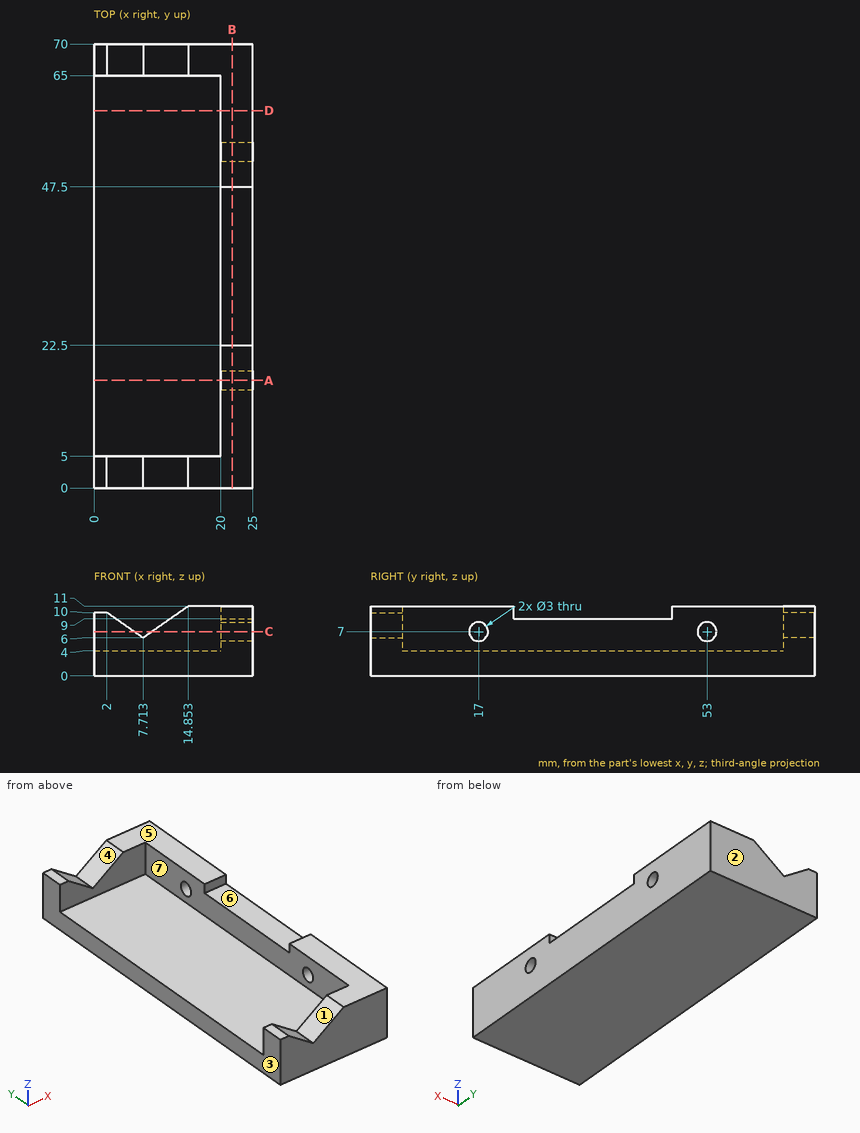
Verification items for this drawing (mm, ordinates from the low corner). A direction names the side the tool comes from. Coordinates: 2 decimals unless noted, no trailing zeros. Write each loop counter-clockwise with the first axis right and the second up, starting at its lowest first coordinate (ties: lowest second). Pieces come first, ordered by that corner, then holes. Notation, with made-up numbers: M 4.5,-18 L 29.5,-18 A30 cw 29.5,12 Z; hole C -22.75,24 d6. An arc over 180 degrees is marked long. One line per item, written item: value. Start each with the question number.
(1) Sectioned sample at A-A, the plane y = 17. Enter the section's corners in (x, z).
(2) Scan lines: line 1 along Y through (x, z) = (21, 7); line 2 along Y through (x, z) = (2.75, 5.5); line 3 along Z through (x, y) = (18.5, 33). Record each from-to range of solid material in increasing order. Write a range as [from, to].
(3) Release check for a two-part mould opening along X. For the marked faces 1, 2, 3 and 4 record: released by +X, released by -X, zero draft, split by the parting line, or undercut.
(4) Sectioned sample at C-C, the plane z = 7. Enter the section's corners in (x, y) (1 decimal).
(5) Sectioned sample at B-B, the plane x = 21.75. Enter the section's corners in (y, z).
(6) Tool access check on the marked faces 5, 6 and 7. Record the directions out of +Z, -Z, +X, -X, +Y, -Y that give a thin tool (end or side, any length) a straight path to the whole face; none if there is none.
(7) Sectioned sample at D-D, the plane y = 59.5. Enter the section's corners in (x, z).
(8) Depth check by flat-ended pin: pin 1 (2 mm diameter, centred on y = 38.5, z = 9, fed in from -X); pin 2 (2 mm diameter, centred on x = 0.5, y = 68, fed in from +Z); pin 3 (3 mm diameter, centred on x = 11, y = 52, fed in from +Z). Enter the tip coordinate at first touch or a pass-through.
Filled sheet:
1. outline: M 0,0 L 25,0 L 25,5.5 L 20,5.5 L 20,4 L 0,4 Z; M 20,8.5 L 25,8.5 L 25,11 L 20,11 Z
2. line 1: [0, 15.5], [18.5, 51.5], [54.5, 70]
2. line 2: [0, 5], [65, 70]
2. line 3: [0, 4]
3. face 1: undercut
3. face 2: zero draft
3. face 3: released by -X
3. face 4: undercut
4. outline: M 0,0 L 6.3,0 L 6.3,5 L 0,5 Z; M 0,65 L 6.3,65 L 6.3,70 L 0,70 Z; M 9.1,0 L 25,0 L 25,15.5 L 20,15.5 L 20,5 L 9.1,5 Z; M 9.1,65 L 20,65 L 20,54.5 L 25,54.5 L 25,70 L 9.1,70 Z; M 20,18.5 L 25,18.5 L 25,51.5 L 20,51.5 Z
5. outline: M 0,0 L 70,0 L 70,11 L 47.5,11 L 47.5,9 L 22.5,9 L 22.5,11 L 0,11 Z; hole C 17,7 d3; hole C 53,7 d3
6. face 5: +Z, +X, -X, +Y, -Y
6. face 6: +Z, +X, -X
6. face 7: +Z, -X
7. outline: M 0,0 L 25,0 L 25,11 L 20,11 L 20,4 L 0,4 Z
8. pin 1: x = 20
8. pin 2: z = 10
8. pin 3: z = 4
